Design review of the part built by this model. Coordinates are the model's own, in mm. A direction names the side the tool comes from. Give positions to 0.01 mm unless a question says otherwise; leave off trailing zeros. Order: outer loops, then holes, each group sorted by start corner. A loop starts at its lowest first (then second) coordinate and runs counter-clockwise, first axis right, second up. Notation, with made-up numbers: (88, 47) -> (127, 47) arc R30 cw to (127, 70) -> close; hole circle Ø7 at (16.25, -28.75). An arc over 180 degrees is marked (long way). Return JSON: item names as keys, results as strings.
```python
from build123d import *

# Parameters (mm, degrees)
SKETCH1_W           = 70
SKETCH1_H           = 155
BOSS_EXTRUDE1_DEPTH = 6
SKETCH3_R           = 15
CUT_EXTRUDE1_DEPTH  = 86.248167136
SKETCH4_R           = 1.75
CUT_EXTRUDE2_DEPTH  = 86.248167136
CUT_EXTRUDE3_DEPTH  = 86.248167136
SKETCH8_R           = 1.75
CUT_EXTRUDE6_DEPTH  = 86.248167136


with BuildPart() as part:
    # Sketch1 → Boss-Extrude1 (new body)
    with BuildSketch(Plane.XY):
        Rectangle(SKETCH1_W, SKETCH1_H)
    extrude(amount=BOSS_EXTRUDE1_DEPTH)

    # Sketch3 → Cut-Extrude1 (cut, through all)
    with BuildSketch(Plane.XY.offset(6)):
        with Locations((0, 42.5)):
            Circle(SKETCH3_R)
    extrude(amount=-CUT_EXTRUDE1_DEPTH, mode=Mode.SUBTRACT)

    # Sketch4 → Cut-Extrude2 (cut, through all)
    with BuildSketch(Plane(origin=(0, 0, 0), x_dir=(-1, 0, 0), z_dir=(0, 0, -1))):
        with Locations((-19, 53.4)):
            Circle(SKETCH4_R)
        with Locations((19, 53.4)):
            Circle(SKETCH4_R)
        with Locations((-19, 15.4)):
            Circle(SKETCH4_R)
        with Locations((19, 15.4)):
            Circle(SKETCH4_R)
    extrude(amount=-CUT_EXTRUDE2_DEPTH, mode=Mode.SUBTRACT)

    # Sketch5 → Cut-Extrude3 (cut, through all)
    with BuildSketch(Plane.XY.offset(6)):
        with BuildLine():
            Line((29.5, 7.5), (31, 7.5))
            ThreePointArc((31, 7.5), (32.060660172, 7.060660172), (32.5, 6))
            Line((32.5, 6), (32.5, -3))
            ThreePointArc((32.5, -3), (32.060660172, -4.060660172), (31, -4.5))
            Line((31, -4.5), (29.5, -4.5))
            ThreePointArc((29.5, -4.5), (28.439339828, -4.060660172), (28, -3))
            Line((28, -3), (28, 6))
            ThreePointArc((28, 6), (28.439339828, 7.060660172), (29.5, 7.5))
        make_face()
    extrude(amount=-CUT_EXTRUDE3_DEPTH, mode=Mode.SUBTRACT)

    # Sketch8 → Cut-Extrude6 (cut, through all)
    with BuildSketch(Plane.XY.offset(6)):
        with Locations((-27.888022688, 42.5)):
            Circle(SKETCH8_R)
        with Locations((0, 14.611977312)):
            Circle(SKETCH8_R)
        with Locations((27.888022688, 42.5)):
            Circle(SKETCH8_R)
        with Locations((0, 70.388022688)):
            Circle(SKETCH8_R)
    extrude(amount=-CUT_EXTRUDE6_DEPTH, mode=Mode.SUBTRACT)


solid = part.part
```
Item 1: Mouldability with a two-part tool opening along X and no side actions: class faces 3 (the face through (-18.772, 55.135, 2.958)), 4 (the face through (35, -1, 3)), 5 (the face through (-0.38, 68.68, 3.04)), 6 (the face through (0, -77.5, 3)) as released by +X, released by -X, zero draft, split by the parting line, or undercut.
Result set:
{"face 3": "undercut", "face 4": "released by +X", "face 5": "undercut", "face 6": "zero draft"}
Item 2: Add section B-B (x = 0). Give the boundary of the cut face in (y, z).
Result set:
{"outline": "(-77.5, 0) -> (12.86, 0) -> (12.86, 6) -> (-77.5, 6) -> close; (16.36, 0) -> (27.5, 0) -> (27.5, 6) -> (16.36, 6) -> close; (57.5, 0) -> (68.64, 0) -> (68.64, 6) -> (57.5, 6) -> close; (72.14, 0) -> (77.5, 0) -> (77.5, 6) -> (72.14, 6) -> close"}
Item 3: Wall thickness on L1, parallel to Y at x = 19, z = 4.85; L2, parallel to Y at x = 0, z = 5.05; L3, parallel to Y at x = 30, z = 0.55: over which ranges is each line inside the solid? List them lowest first. Write a range as [from, to].
Result set:
{"L1": "y = [-77.5, 13.65], [17.15, 51.65], [55.15, 77.5]", "L2": "y = [-77.5, 12.86], [16.36, 27.5], [57.5, 68.64], [72.14, 77.5]", "L3": "y = [-77.5, -4.5], [7.5, 77.5]"}
Item 4: Add section C-C (x = -19). Give the boundary of the cut face in (y, z).
Result set:
{"outline": "(-77.5, 0) -> (13.65, 0) -> (13.65, 6) -> (-77.5, 6) -> close; (17.15, 0) -> (51.65, 0) -> (51.65, 6) -> (17.15, 6) -> close; (55.15, 0) -> (77.5, 0) -> (77.5, 6) -> (55.15, 6) -> close"}
Item 5: Add section D-D (x = 7). Give the boundary of the cut face in (y, z), plus the area to 3 significant figures.
Result set:
{"outline": "(-77.5, 0) -> (29.23, 0) -> (29.23, 6) -> (-77.5, 6) -> close; (55.77, 0) -> (77.5, 0) -> (77.5, 6) -> (55.77, 6) -> close", "area": "771 mm^2"}
Item 6: Machinability: for faces 1 (the face through (28, 1, 3)), 2 (the face through (0, 77.5, 3)), which of the approach directions +Z, -Z, +X, -X, +Y, -Y give a long, thin tool a straight path to every point of the face, cutting with its end or side? Answer none if there is none.
Result set:
{"face 1": "+Z, -Z", "face 2": "+Z, -Z, +X, -X, +Y"}
Item 7: Add section A-A (y = 42.5). Give the boundary of the cut face in (x, z), plus the area to 3 significant figures.
Result set:
{"outline": "(-35, 0) -> (-29.64, 0) -> (-29.64, 6) -> (-35, 6) -> close; (-26.14, 0) -> (-15, 0) -> (-15, 6) -> (-26.14, 6) -> close; (15, 0) -> (26.14, 0) -> (26.14, 6) -> (15, 6) -> close; (29.64, 0) -> (35, 0) -> (35, 6) -> (29.64, 6) -> close", "area": "198 mm^2"}
